Design review of the part built by this model. Coordinates are the model's own, in mm. A direction names the side the tool comes from. Coordinates: 2 decimals unless noted, no trailing zeros. Loops run counter-clockwise (first coordinate to the right, second up) from the corner with the lowest first, then second, coordinate; pieces in that order, holes last. Notation, with made-up numbers: M 84.25,58.5 L 92.25,58.5 A21 cw 92.25,85.5 Z; hole C 9,78.5 d9. An arc over 180 degrees is marked long. Put each result on its own line as item: value. Start each with the question number.
(1) Take a section at C-C, the plane z = 3.5. Count the separate pieces of the cut face and the enclosed holes in it, then the cut area to 3 significant figures.
(2) For faces 1 (the cylindrical face through (-12.283, 8.496, 2.638)), 2 (the flat face through (4, 5, 6.35)), 3 (the cylindrical face through (11.01, -7.87, 6.87)), list the 3-axis set-ups (+Z, -Z, +X, -X, +Y, -Y) from which the entire face can be reached by the end or side of a thin tool; tool diameter is ignored.
(3) The part is to be moulded in two halves that separate along X. For faces 4 (the flat face through (4, 0, 8.35)), 5 (the cylindrical face through (11.76, 9.93, 6.87)), say which applies: +X half, -X half, draft (parallel to the pull), parting line (faces both ways), or undercut.
(4) For probe 1 along X at (y, z) = (-9, 5.25); probe 2 along X at (y, z) = (10, 8.25); probe 3 along Y at (x, z) = (0, 3.5), list the stretches that pass through material, from the lowest coordinate up. Write a range as [from, to].
(5) Clearance check with flat-ended pins moving along their axes: pin 1 (3 mm diameter, centred on x = 14.5, y = -9, fed in from +Z); pin 2 (7.5 mm diameter, centred on x = -13.86, y = -8, fed in from -Z); pin 3 (1.5 mm diameter, centred on x = 10.5, z = 3.5, fed in from +Y). State where each tip first meets the part, or that it passes through.
(6) Take a section at B-B, the plane x = 0. Give the boundary of the cut face in (y, z).
(7) Take a section at D-D, the plane y = 2.25. Give the boundary of the cut face in (x, z), then the cut area to 3 significant figures.
(8) Take a section at A-A, the plane z = 7.5. Give the boundary of the cut face in (x, y).
```python
from build123d import *
from build123d.topology import SkipClean

# Parameters (mm, degrees)
SKETCH1_R             = 3.35
SKETCH1_R_2           = 1.65
BOSS_EXTRUDE1_DEPTH   = 6.35
BOSS_EXTRUDE1_2_DEPTH = 6.35
BOSS_EXTRUDE1_3_DEPTH = 6.35
BOSS_EXTRUDE1_4_DEPTH = 6.35
SKETCH1_R_3           = 6
SKETCH1_R_4           = 3.45
BOSS_EXTRUDE1_5_DEPTH = 6.35
SKETCH2_R             = 1.65
SKETCH2_R_2           = 6
SKETCH2_R_3           = 3.45
BOSS_EXTRUDE2_DEPTH   = 2
SKETCH3_R             = 2.85
CUT_EXTRUDE1_DEPTH    = 3


with BuildPart() as part:
    # Sketch1 → Boss-Extrude1 (new body)
    with BuildSketch(Plane.XY):
        with Locations((-13.856406461, 8)):
            Circle(SKETCH1_R)
        with Locations((-13.856406461, 8)):
            Circle(SKETCH1_R_2, mode=Mode.SUBTRACT)
    extrude(amount=BOSS_EXTRUDE1_DEPTH)



with BuildPart() as body_2:
    # Sketch1 → Boss-Extrude1 2 (new body)
    with BuildSketch(Plane.XY):
        with Locations(Location((-13.856406461, -8, 0), (0, 0, 180))):
            Circle(SKETCH1_R)
        with Locations(Location((-13.856406461, -8, 0), (0, 0, 180))):
            Circle(SKETCH1_R_2, mode=Mode.SUBTRACT)
    extrude(amount=BOSS_EXTRUDE1_2_DEPTH)


with BuildPart() as body_3:
    # Sketch1 → Boss-Extrude1 3 (new body)
    with BuildSketch(Plane.XY):
        with Locations((13.856406461, -8)):
            Circle(SKETCH1_R)
        with Locations((13.856406461, -8)):
            Circle(SKETCH1_R_2, mode=Mode.SUBTRACT)
    extrude(amount=BOSS_EXTRUDE1_3_DEPTH)


with BuildPart() as body_4:
    # Sketch1 → Boss-Extrude1 4 (new body)
    with BuildSketch(Plane.XY):
        with Locations(Location((13.856406461, 8, 0), (0, 0, 180))):
            Circle(SKETCH1_R)
        with Locations(Location((13.856406461, 8, 0), (0, 0, 180))):
            Circle(SKETCH1_R_2, mode=Mode.SUBTRACT)
    extrude(amount=BOSS_EXTRUDE1_4_DEPTH)


with BuildPart() as body_5:
    # Sketch1 → Boss-Extrude1 5 (new body)
    with BuildSketch(Plane.XY):
        Circle(SKETCH1_R_3)
        Circle(SKETCH1_R_4, mode=Mode.SUBTRACT)
    extrude(amount=BOSS_EXTRUDE1_5_DEPTH)


with BuildPart() as part_1:
    with SkipClean():  # the faces are left unmerged after this step: merging them gives an invalid solid
        add(part.part)

        add(body_2.part)  # Boss-Extrude2 merges body 2

        add(body_3.part)  # Boss-Extrude2 merges body 3

        add(body_4.part)  # Boss-Extrude2 merges body 4

        add(body_5.part)  # Boss-Extrude2 merges body 5
        # Sketch2 → Boss-Extrude2 (add)
        # profile 1 of 2: a face of its own
        with BuildSketch(Plane.XY.offset(6.35)):
            with BuildLine():
                Line((-13.856406461, 11.35), (13.856406461, 11.35))
                ThreePointArc((13.856406461, 11.35), (16.225214178, 10.368807717), (17.206406461, 8))
                Line((17.206406461, 8), (17.206406461, -8))
                ThreePointArc((17.206406461, -8), (16.225214178, -10.368807717), (13.856406461, -11.35))
                Line((13.856406461, -11.35), (-13.856406461, -11.35))
                ThreePointArc((-13.856406461, -11.35), (-16.225214178, -10.368807717), (-17.206406461, -8))
                Line((-17.206406461, -8), (-17.206406461, 8))
                ThreePointArc((-17.206406461, 8), (-16.225214178, 10.368807717), (-13.856406461, 11.35))
            make_face()
            with Locations((-13.856406461, 8)):
                Circle(SKETCH2_R, mode=Mode.SUBTRACT)
            with Locations(Location((-13.856406461, -8, 0), (0, 0, 180))):
                Circle(SKETCH2_R, mode=Mode.SUBTRACT)
            with Locations(Location((13.856406461, 8, 0), (0, 0, 180))):
                Circle(SKETCH2_R, mode=Mode.SUBTRACT)
            with Locations((13.856406461, -8)):
                Circle(SKETCH2_R, mode=Mode.SUBTRACT)
            Circle(SKETCH2_R_2, mode=Mode.SUBTRACT)
        # profile 2 of 2: a face of its own
        with BuildSketch(Plane.XY.offset(6.35)):
            Circle(SKETCH2_R_2)
            Circle(SKETCH2_R_3, mode=Mode.SUBTRACT)
        extrude(amount=BOSS_EXTRUDE2_DEPTH)

    # Sketch3 → Cut-Extrude1 (cut)
    with SkipClean():  # the faces are left unmerged after this step: merging them gives an invalid solid
        with BuildSketch(Plane.XY.offset(8.35)):
            with Locations((-13.856406461, 8)):
                Circle(SKETCH3_R)
            with Locations((-13.856406461, -8)):
                Circle(SKETCH3_R)
            with Locations((13.856406461, -8)):
                Circle(SKETCH3_R)
            with Locations((13.856406461, 8)):
                Circle(SKETCH3_R)
        extrude(amount=-CUT_EXTRUDE1_DEPTH, mode=Mode.SUBTRACT)


solid = part_1.part
```
Computed values:
1. separate pieces: 5
1. enclosed holes: 5
1. area: 183 mm^2
2. face 1: +Z, -Z
2. face 2: -Z
2. face 3: +Z
3. face 4: draft
3. face 5: undercut
4. probe 1: x = [-17.05, -15.17], [-12.54, -10.66], [10.66, 12.54], [15.17, 17.05]
4. probe 2: x = [-16.54, -15.89], [-11.83, 11.83], [15.89, 16.54]
4. probe 3: y = [-6, -3.45], [3.45, 6]
5. pin 1: stops at z = 5.35
5. pin 2: stops at z = 0
5. pin 3: stops at y = 10.1
6. outline: M -11.35,6.35 L -6,6.35 L -6,0 L -3.45,0 L -3.45,8.35 L -11.35,8.35 Z; M 3.45,0 L 6,0 L 6,6.35 L 11.35,6.35 L 11.35,8.35 L 3.45,8.35 Z
7. outline: M -17.21,6.35 L -5.56,6.35 L -5.56,0 L -2.62,0 L -2.62,8.35 L -17.21,8.35 Z; M 2.62,0 L 5.56,0 L 5.56,6.35 L 17.21,6.35 L 17.21,8.35 L 2.62,8.35 Z
7. area: 95.8 mm^2
8. outline: M -17.21,-8 A3.35 ccw -13.86,-11.35 L 13.86,-11.35 A3.35 ccw 17.21,-8 L 17.21,8 A3.35 ccw 13.86,11.35 L -13.86,11.35 A3.35 ccw -17.21,8 Z; hole C -13.86,-8 d5.7; hole C -13.86,8 d5.7; hole C 0,0 d6.9; hole C 13.86,-8 d5.7; hole C 13.86,8 d5.7
